```python
from build123d import *

# Parameters (mm, degrees)
SKETCH1_R           = 4.75
SKETCH1_R_2         = 3.001
BOSS_EXTRUDE1_DEPTH = 4
SKETCH2_R           = 6
SKETCH2_R_2         = 3.001
BOSS_EXTRUDE2_DEPTH = 1
SCALE1_SCALE        = 1.5


with BuildPart() as part:
    # Sketch1 → Boss-Extrude1 (new body)
    with BuildSketch(Plane(origin=(0, 0, 0), x_dir=(1, 0, 0), z_dir=(0, 1, 0))):
        Circle(SKETCH1_R)
        Circle(SKETCH1_R_2, mode=Mode.SUBTRACT)
    extrude(amount=BOSS_EXTRUDE1_DEPTH)

    # Sketch2 → Boss-Extrude2 (add)
    with BuildSketch(Plane.XZ):
        Circle(SKETCH2_R)
        Circle(SKETCH2_R_2, mode=Mode.SUBTRACT)
    extrude(amount=BOSS_EXTRUDE2_DEPTH)


with BuildPart() as part_1:
    # Scale1: scaled about (0, 1.169108574, 0)
    add(part.part.scale(SCALE1_SCALE).moved(Location((0, -0.584554287, 0))))


solid = part_1.part
```
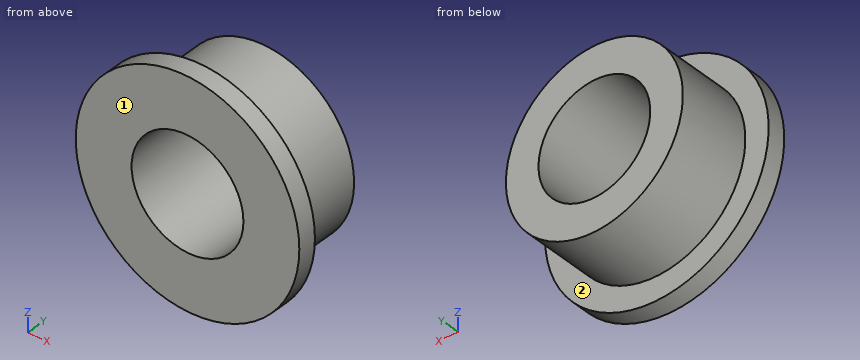
Could you check a few things on this model? Use its own coordinates, in mm. Face numbers are marked on the shaded views. A direction names the side the tool comes from. Round coordinates to 2 decimals unless told otherwise and drop trailing zeros. Write each loop counter-clockwise with the first axis right and the second up, starting at its lowest first coordinate (ties: lowest second). Pieces come first, ordered by that corner, then holes. Notation, with made-up numbers: M -38,34.5 L -23,34.5 A27 cw -23,57.5 Z; hole C 52,85.25 d5. An arc over 180 degrees is marked long. Write each question's results on one line, items separated by ' | '. Start each with the question number.
1. I need wall thicknesses on L1, parallel to Z at x = 0, y = 0 (1 decimal); L2, parallel to Z at x = 0, y = -1. Which ranges of each line are inside material? Lowest first, please. Write a range as from..to.
2. Imagine slicing it at A-A on z = 0. List the corners of the cut face in (x, y) for me (1 decimal), and give its area (3 significant figures).
3. Imagine slicing it at B-B on x = 0. List the corners of the cut face in (y, z) for me (1 decimal), and give its area (3 significant figures).
4. On a 3-axis mill with a long thin cutter (end or side, diameter ignored), from which of +Z, -Z, +X, -X, +Y, -Y can I reach the whole of each face in a straight line? I mean the marked faces 1 and 2. Say none if no direction works.
5. Imagine slicing it at D-D on x = -5.5. List the corners of the cut face in (y, z) for me, and give its area (3 significant figures).
6. I'm going to push flat-ended pins straight in: pin 1 Ø2 at (x, y) = (-0.5, 3) entering from -Z (3 decimals); pin 2 Ø1 at (x, y) = (5, -1) entering from -Z; pin 3 Ø8 at (x, z) = (1.5, -3) entering from -Y; pin 4 Ø1.5 at (x, y) = (-3, -1) entering from -Z. Where does each tip first touch, or does it pass through?
Result sheet:
1) L1: z = -7.1..-4.5, 4.5..7.1 | L2: z = -9..-4.5, 4.5..9
2) outline: M -9,-2.1 L -4.5,-2.1 L -4.5,5.4 L -7.1,5.4 L -7.1,-0.6 L -9,-0.6 Z; M 4.5,-2.1 L 9,-2.1 L 9,-0.6 L 7.1,-0.6 L 7.1,5.4 L 4.5,5.4 Z | area: 45.0 mm^2
3) outline: M -2.1,-9 L -0.6,-9 L -0.6,-7.1 L 5.4,-7.1 L 5.4,-4.5 L -2.1,-4.5 Z; M -2.1,4.5 L 5.4,4.5 L 5.4,7.1 L -0.6,7.1 L -0.6,9 L -2.1,9 Z | area: 45.0 mm^2
4) face 1: +Z, -Z, +X, -X, -Y | face 2: +Y
5) outline: M -2.08,-7.12 L -0.58,-7.12 L -0.58,-4.53 L 5.42,-4.53 L 5.42,4.53 L -0.58,4.53 L -0.58,7.12 L -2.08,7.12 Z | area: 75.7 mm^2
6) pin 1: stops at z = -7.125 | pin 2: stops at z = -7.79 | pin 3: stops at y = -2.08 | pin 4: stops at z = -8.71
